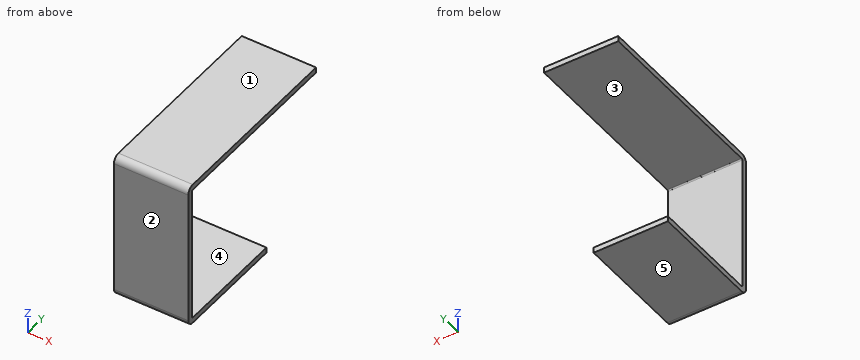
Autodesk Inventor part; units mm, degrees
ref_plane "YZ Plane" through (0, 0, 0) normal (1, 0, 0) x (0, 1, 0)
ref_plane "XZ Plane" through (0, 0, 0) normal (0, 1, 0) x (-1, 0, 0)
ref_plane "XY Plane" through (0, 0, 0) normal (0, 0, 1) x (1, 0, 0)
sketch "Sketch1" plane through (0, 0, 0) normal (0, 1, 0) x (-1, 0, 0)
  line L0 (10, -18.5) -> (-10, -18.5)
  line L1 (-10, -18.5) -> (-10, 18.5)
  line L2 (-10, 18.5) -> (10, 18.5)
  line L3 (10, 18.5) -> (10, -18.5)
  point P0 (0, 0)
  dimension "d0" = 20
  dimension "d1" = 37
  dimension "d2" = 18.5
  dimension "d3" = 10
extrude "Plate1" add sketch "Sketch1" along normal blind 1.5
sketch "Sketch2" plane through (-10, 0, -20) normal (0, 0, 1) x (1, 0, 0)
  line L0 (20, 0) -> (0, 0)
  line L1 (0, 0) -> (0, 31.5)
  line L2 (0, 31.5) -> (20, 31.5)
  line L3 (20, 31.5) -> (20, 0)
edge flange "Flange1" height 31.5 angle 90 thickness 1.5 bend radius 0.31 thickness toward (0, 0, 1) relief tear relief width 1.5 relief depth 0.75 edges at (0, 1.5, -18.5) wall of the first edge with corners at (10, 0, -20) (-10, 0, -20) (-10, 31.5, -20) (10, 31.5, -20)
bend "Bend1"
corner "Corner1"
sketch "Sketch3" plane through (10, 0, 20) normal (0, 0, -1) x (-1, 0, 0)
  line L0 (20, 0) -> (0, 0)
  line L1 (0, 0) -> (0, 51.5)
  line L2 (0, 51.5) -> (20, 51.5)
  line L3 (20, 51.5) -> (20, 0)
edge flange "Flange2" height 51.5 angle 90 thickness 1.5 bend radius 0.31 thickness toward (0, 0, -1) relief tear relief width 1.5 relief depth 0.75 edges at (0, 1.5, 18.5) wall of the first edge with corners at (-10, 0, 20) (10, 0, 20) (10, 51.5, 20) (-10, 51.5, 20)
bend "Bend2"
corner "Corner2"
equation "\"d4\" = Thickness"
equation "\"d5\" = BendReliefWidth"
equation "\"d6\" = BendReliefDepth"
equation "\"d7\" = MinimumRemnant"
equation "\"d8\" = TransitionRadius"
equation "\"d11\" = BendRadius"
equation "\"d12\" = CornerReliefSize"
equation "\"d13\" = GapSize"
equation "\"d14\" = JacobiRadiusSize"
equation "\"d15\" = BendReliefWidth"
equation "\"d16\" = BendReliefDepth"
equation "\"d17\" = MinimumRemnant"
equation "\"d18\" = TransitionRadius"
equation "\"d21\" = BendRadius"
equation "\"d22\" = CornerReliefSize"
equation "\"d23\" = GapSize"
equation "\"d24\" = JacobiRadiusSize"
equation "\"BendReliefWidth\" = Thickness"
equation "\"BendReliefDepth\" = 0.5 * Thickness"
equation "\"CornerReliefSize\" = 4 * Thickness"
equation "\"MinimumRemnant\" = 2 * Thickness"
equation "\"TransitionRadius\" = BendRadius"
equation "\"JacobiRadiusSize\" = BendRadius"
equation "\"GapSize\" = Thickness"
properties part number "axis_9_bottom_frame" material "Aluminum 6061-AHC"
Work out the finished part from the listing and answer in its coordinate system (mm). Face numbers are marked on the shaded views. A direction names the side the tool comes from. Give positions to 0.01 mm unless a question says otherwise; leave off trailing zeros. Loops run counter-clockwise (first coordinate to the right, second up) from the corner with the lowest first, then second, coordinate; pieces in that order, holes last. Notation, with made-up numbers: (65.5, -4) -> (120.5, -4) arc R30 cw to (120.5, 31) -> close; hole circle Ø8 at (33.25, 86). An arc over 180 degrees is marked (long way). One line per question, with ' | ' between items. Start each with the question number.
1) Straight lines are drawn through the part: L1, parallel to Z at x = 0, y = 31; L2, parallel to Y at x = -2.75, z = -5.5; L3, parallel to Z at x = -3.5, y = 33. For each, find the intervals that lie inside material, in ascending order.
2) Section C-C, the plane z = 2.5 is taken. Determine the outline of the cut face in (x, y), then the cut area to 3 significant figures.
3) Section B-B, the plane x = 0.75 is taken. Determine the outline of the cut face in (y, z).
4) Determine the mould class of the marked faces 1, 2 and 3 for opening direction Z: +Z half, -Z half, draft (parallel to the pull), parting line (faces both ways), or undercut.
5) Each of these flat-tipped pins is pushed along its axis until it touches: pin 1 (1 mm diameter, centred on x = -5, z = -2.5, fed in from +Y); pin 2 (1.6 mm diameter, centred on x = -2.5, z = -19.5, fed in from +Y). Where does it stop, or does it pass through?
6) For the marked faces 4 and 5, determine the directions among +Z, -Z, +X, -X, +Y, -Y from which every point of the face is accessible in a straight line to the end or side of a thin tool.
7) Section A-A, the plane y = 7 is taken. Determine the outline of the cut face in (x, z).
8) Section D-D, the plane y = 37 is taken. Determine the outline of the cut face in (x, z), then the cut area to 3 significant figures.
Resolved:
1) L1: -20 to -18.5, 18.5 to 20 | L2: 0 to 1.5 | L3: 18.5 to 20
2) outline: (-10, 0) -> (10, 0) -> (10, 1.5) -> (-10, 1.5) -> close | area: 30.0 mm2
3) outline: (0, -18.19) arc R1.81 ccw to (1.81, -20) -> (31.5, -20) -> (31.5, -18.5) -> (1.81, -18.5) arc R0.31 cw to (1.5, -18.19) -> (1.5, 18.19) arc R0.31 cw to (1.81, 18.5) -> (51.5, 18.5) -> (51.5, 20) -> (1.81, 20) arc R1.81 ccw to (0, 18.19) -> close
4) face 1: +Z half | face 2: draft | face 3: undercut
5) pin 1: y = 1.5 | pin 2: y = 31.5
6) face 4: +X, -X, +Y | face 5: -Z, +X, -X, +Y, -Y
7) outline: (-10, -20) -> (10, -20) -> (10, -18.5) -> (-10, -18.5) -> close; (-10, 18.5) -> (10, 18.5) -> (10, 20) -> (-10, 20) -> close
8) outline: (-10, 18.5) -> (10, 18.5) -> (10, 20) -> (-10, 20) -> close | area: 30.0 mm2
